Read the model definition and answer for the solid it produces. Units are mm, in the model's axes. A direction names the side the tool comes from. Give positions to 0.01 mm unless a question says otherwise; leave off trailing zeros. Write each loop counter-clockwise with the first axis right and the second up, starting at its lowest first coordinate (ties: lowest second). Pieces come first, ordered by that corner, then holes. Notation, with made-up numbers: M -5,71.25 L 1,71.25 A24 ccw 1,104.25 Z; hole C -39.75,29 d1. An arc over 180 degrees is marked long. Put each result on its own line as item: value.
from build123d import *

# Parameters (mm, degrees)
ESQUISSE1_W             = 90
ESQUISSE1_H             = 40
BOSS_EXTRU_1_DEPTH      = 45
ENL_V_MAT_EXTRU_2_DEPTH = 45
ENL_V_MAT_EXTRU_3_DEPTH = 106
ESQUISSE6_R             = 12.5
ENL_V_MAT_EXTRU_4_DEPTH = 25
ESQUISSE7_R             = 5
ENL_V_MAT_EXTRU_5_DEPTH = 56
ESQUISSE9_R             = 2
ENL_V_MAT_EXTRU_6_DEPTH = 11


with BuildPart() as part:
    # Esquisse1 → Boss.-Extru.1 (new body)
    with BuildSketch(Plane.XY):
        Rectangle(ESQUISSE1_W, ESQUISSE1_H)
    extrude(amount=BOSS_EXTRU_1_DEPTH)

    # Esquisse2 → Enlèv. mat.-Extru.2 (cut)
    with BuildSketch(Plane.XZ.offset(20)):
        Polygon((45, 45), (12.5, 45), (45, 30.113476392), align=None)
        Polygon((-45, 30.113476392), (-12.5, 45), (-45, 45), align=None)
    extrude(amount=-ENL_V_MAT_EXTRU_2_DEPTH, mode=Mode.SUBTRACT)

    # Esquisse3 → Enlèv. mat.-Extru.3 (cut)
    with BuildSketch(Plane(origin=(45, 0, 0), x_dir=(0, 0, -1), z_dir=(1, 0, 0))):
        Polygon((0, -20), (-10.965276347, 20), (0, 20), align=None)
        Polygon((-45, 0), (-39.517361826, -20), (-45, -20), align=None)
    extrude(amount=-ENL_V_MAT_EXTRU_3_DEPTH, mode=Mode.SUBTRACT)

    # Esquisse6 → Enlèv. mat.-Extru.4 (cut)
    with BuildSketch(Plane(origin=(19.205292649, 0, 41.928661621), x_dir=(0.90916344, 0, -0.416439478), z_dir=(0.416439478, 0, 0.90916344))):
        with Locations((10.771914446, 0)):
            Circle(ESQUISSE6_R)
    enl_v_mat_extru_4 = extrude(amount=-ENL_V_MAT_EXTRU_4_DEPTH, mode=Mode.SUBTRACT)

    # Symétrie1: Enlèv. mat.-Extru.4 across plane
    add(enl_v_mat_extru_4.mirror(Plane(origin=(0, 0, 0), x_dir=(0, 0, 1), z_dir=(1, 0, 0))), mode=Mode.SUBTRACT)

    # Esquisse7 → Enlèv. mat.-Extru.5 (cut)
    with BuildSketch(Plane(origin=(0, -11.473706327, 41.854690985), x_dir=(1, 0, 0), z_dir=(0, -0.264378055, 0.964419123))):
        with Locations((0, 1.6591408)):
            Circle(ESQUISSE7_R)
    extrude(amount=-ENL_V_MAT_EXTRU_5_DEPTH, mode=Mode.SUBTRACT)

    # Esquisse9 → Enlèv. mat.-Extru.6 (cut)
    with BuildSketch(Plane(origin=(0, -1.397915118, 5.099425034), x_dir=(-1, 0, 0), z_dir=(0, 0.264378055, -0.964419123))):
        with Locations((35, 1.496078457)):
            Circle(ESQUISSE9_R)
        with Locations((-35, 1.822203143)):
            Circle(ESQUISSE9_R)
    extrude(amount=-ENL_V_MAT_EXTRU_6_DEPTH, mode=Mode.SUBTRACT)


solid = part.part
(1) Section C-C on z = 22 is taken. Give the number of separate pieces and of enclosed holes in the cut face, and give its area (3 significant figures).
Result:
separate pieces: 1
enclosed holes: 3
area: 2,440 mm²
(2) Which of the six approach directions +Z, -Z, +X, -X, +Y, -Y give full straight-line access (tool end or side, diameter ignored) to faces 5 (the face through (0, 10, 45)), 6 (the face through (18.4, 0.2, 14.8))?
Result:
face 5: +Z, +X, -X, +Y, -Y
face 6: none
(3) Section B-B on x = 0 is taken. Determine the outline of the cut face in (y, z).
Result:
outline: M -20,0 L -4.62,4.22 L -14.7,40.97 L -20,39.52 Z; M -5.05,43.62 L 5.02,6.86 L 20,10.97 L 20,45 L 0,45 Z
(4) Straight lines are drawn through the part: line 1 along X through (y, z) = (1, 32); line 2 along X through (y, z) = (-3.5, 21); line 3 along X through (y, z) = (7.5, 12). For each, find the intervals that lie inside material, in ascending order. Write a range as from..to.
Result:
line 1: x = -40.88..-40.21, -12.8..12.8, 40.21..40.88
line 2: x = -45..-34.67, -8.27..-4.97, 4.97..8.27, 34.67..45
line 3: x = -45..-28.34, -24.51..24.51, 28.34..45
(5) Section D-D on y = 16.5 is taken. Determine the outline of the cut face in (x, z).
Result:
outline: M -45,10.01 L 45,10.01 L 45,30.11 L 12.5,45 L -12.5,45 L -45,30.11 Z
(6) For a pull along Z with two mould halves and no side action, classify faces 1 (the face through (28.52, 13.05, 37.66)), 2 (the face through (0.63, -9.17, 2.97)), 3 (the face through (34.706, 3.755, 21.272)), 4 (the face through (-45, 0, 18)) as +Z half, -Z half, draft (parallel to the pull), parting line (faces both ways), or undercut.
Result:
face 1: +Z half
face 2: -Z half
face 3: undercut
face 4: draft
(7) Given pin 1 Ø12 at (x, y) = (26, 14) entering from -Z, flat-ended and moving along its own axis, determine where the tip first touches the part or whether it passes through.
Result:
pin 1: stops at z = 7.68
(8) Section A-A on y = 6 is taken. Determine the outline of the cut face in (x, z).
Result:
outline: M -45,7.13 L 45,7.13 L 45,30.11 L 38.97,32.88 L 28.56,10.15 L 8.62,19.28 L 19.03,42.01 L 12.5,45 L -12.5,45 L -19.03,42.01 L -8.62,19.28 L -28.56,10.15 L -38.97,32.88 L -45,30.11 Z
